Read the model definition and answer for the solid it produces. Units are mm, in the model's axes. A direction names the side the tool comes from. Coordinates: 2 decimals unless noted, no trailing zeros. Loops run counter-clockwise (first coordinate to the right, second up) from the corner with the lowest first, then second, coordinate; pieces in that order, holes last. Notation, with made-up numbers: (49, 28) - (103, 28) arc R20 ccw to (103, 51) - close; hole circle Ø10 at (-18, -8.5). An arc over 180 degrees is marked (long way). One line per question, with ' | ' between items. Start each with the question number.
```python
from build123d import *

# Parameters (mm, degrees)
F0_R     = 13
F1_DEPTH = 94
F2_R     = 13
F2_R_2   = 7.5
F3_DEPTH = 15
F4_R     = 13
F4_R_2   = 7.5
F5_DEPTH = 49


with BuildPart() as f1:
    # F0 (on Front) → F1 (new body)
    with BuildSketch(Plane.XZ):
        Circle(F0_R)
    extrude(amount=F1_DEPTH)

    # F2 (on face) → F3 (cut)
    with BuildSketch(Plane.XZ.offset(94)):
        Circle(F2_R)
        Circle(F2_R_2, mode=Mode.SUBTRACT)
    extrude(amount=-F3_DEPTH, mode=Mode.SUBTRACT)

    # F4 (on face) → F5 (cut)
    with BuildSketch(Plane(origin=(0, 0, 0), x_dir=(-1, 0, 0), z_dir=(0, 1, 0))):
        Circle(F4_R)
        Circle(F4_R_2, mode=Mode.SUBTRACT)
    extrude(amount=-F5_DEPTH, mode=Mode.SUBTRACT)


solid = f1.part
```
1) Which of the six approach directions +Z, -Z, +X, -X, +Y, -Y give full straight-line access (tool end or side, diameter ignored) to faces 3 (the cylindrical face through (7.493, -24.157, 0.33)), 4 (the flat face through (6, -79, -6)), 5 (the flat face through (0, -94, 0))?
2) The part is cut by section B-B on x = 0. Write down the section's boundary in (y, z).
3) Find the intervals of material crossed by line 1 along Y through (x, z) = (-9, -4.25); line 2 along X through (y, z) = (-89, 1.75), in increasing order. Write a range as from..to.
4) Given pin 1 Ø1.5 at (y, z) = (-17.5, -0.5) entering from -X; pin 2 Ø3 at (x, z) = (6, -8.5) entering from +Y; pin 3 Ø10 at (x, z) = (-5.5, -7) entering from -Y; pin 4 Ø2 at (x, z) = (-9, -3) entering from -Y, each flat-ended and moving along its own axis, determine where each tip first touches the part or whether it passes through.
5) The part is cut by section C-C on y = -85.5. Write down the section's boundary in (x, z).
6) The mould has two halves that part along X. Classify faces 1 (the cylindrical face through (-7.493, -86.605, 0.33)), 2 (the flat face through (-6, -49, -6)): released by +X, released by -X, zero draft, split by the parting line, or undercut.
7) The part is cut by section D-D on y = -62. Write down the section's boundary in (x, z), and give its area (3 significant figures).
8) The part is cut by section A-A on z = 0. Write down the section's boundary in (x, y), and give its area (3 significant figures).
Answer below:
1) face 3: +Y | face 4: -Y | face 5: +Z, -Z, +X, -X, -Y
2) outline: (-94, -7.5) - (-79, -7.5) - (-79, -13) - (-49, -13) - (-49, -7.5) - (0, -7.5) - (0, 7.5) - (-49, 7.5) - (-49, 13) - (-79, 13) - (-79, 7.5) - (-94, 7.5) - close
3) line 1: -79..-49 | line 2: -7.29..7.29
4) pin 1: x = -7.5 | pin 2: y = -49 | pin 3: y = -94 | pin 4: y = -79
5) outline: circle Ø15 at (0, 0)
6) face 1: split by the parting line | face 2: zero draft
7) outline: circle Ø26 at (0, 0) | area: 531 mm2
8) outline: (-13, -79) - (-7.5, -79) - (-7.5, -94) - (7.5, -94) - (7.5, -79) - (13, -79) - (13, -49) - (7.5, -49) - (7.5, 0) - (-7.5, 0) - (-7.5, -49) - (-13, -49) - close | area: 1,740 mm2
